from build123d import *

# Parameters (mm, degrees)
EXTRUDE_1_DEPTH         = 12
SKETCH_5_R              = 33
SKETCH_5_R_2            = 10
CUT_EXTRUDE_1_DEPTH     = 349.001436779
CUT_EXTRUDE_2_DEPTH     = 349.001436779
FILLET_1_R              = 2
HOLE_WIZARD_3_2_3_2_1_D = 3.2


with BuildPart() as part:
    # 草图1 → 凸台-拉伸1 (new body)
    with BuildSketch(Plane.XY):
        with BuildLine():
            Line((320, 25), (56.665686266, 25))
            ThreePointArc((56.665686266, 25), (40.770417333, 27.593877763), (26.524363784, 35.106382979))
            ThreePointArc((26.524363784, 35.106382979), (-44, 0), (26.524363784, -35.106382979))
            ThreePointArc((26.524363784, -35.106382979), (40.770417333, -27.593877763), (56.665686266, -25))
            Line((56.665686266, -25), (320, -25))
            ThreePointArc((320, -25), (345, 0), (320, 25))
        make_face()
    extrude(amount=EXTRUDE_1_DEPTH)

    # 草图5 → 切除-拉伸1 (cut, through all)
    with BuildSketch(Plane.XY.offset(12)):
        Circle(SKETCH_5_R)
        with Locations((320, 0)):
            Circle(SKETCH_5_R_2)
    extrude(amount=-CUT_EXTRUDE_1_DEPTH, mode=Mode.SUBTRACT)

    # 草图6 → 切除-拉伸2 (cut, through all)
    with BuildSketch(Plane.XY.offset(12)):
        with BuildLine():
            Line((112.915026221, 15), (82.915026221, -15))
            Line((82.915026221, -15), (72.915026221, -15))
            Line((72.915026221, -15), (52.915026221, -15))
            ThreePointArc((52.915026221, -15), (55, 0), (52.915026221, 15))
            Line((52.915026221, 15), (112.915026221, 15))
        make_face()
        Polygon((97.057161845, -15), (174.604308358, -15), (127.057161845, 15), align=None)
        Polygon((145.797288554, 15), (212.27301577, 15), (193.344435067, -15), align=None)
        Polygon((205.168568427, -15), (224.097149131, 15), (265.168568427, -15), align=None)
        with BuildLine():
            Line((241.050881866, 15), (282.122301163, -15))
            Line((282.122301163, -15), (300, -15))
            ThreePointArc((300, -15), (295, 0), (300, 15))
            Line((300, 15), (241.050881866, 15))
        make_face()
    extrude(amount=-CUT_EXTRUDE_2_DEPTH, mode=Mode.SUBTRACT)

    # 圆角1
    fillet_1_edges = [part.edges().sort_by_distance(p)[0] for p in [
        (97.057161845, -15, 6),
        (127.057161845, 15, 6),
        (174.604308358, -15, 6),
        (82.915026221, -15, 6),
        (52.915026221, -15, 6),
        (52.915026221, 15, 6),
        (112.915026221, 15, 6),
        (193.344435067, -15, 6),
        (145.797288554, 15, 6),
        (212.27301577, 15, 6),
        (241.050881866, 15, 6),
        (300, 15, 6),
        (300, -15, 6),
        (282.122301163, -15, 6),
        (265.168568427, -15, 6),
        (205.168568427, -15, 6),
        (224.097149131, 15, 6),
    ]]
    fillet(fillet_1_edges, radius=FILLET_1_R)

    # Ø3.2 (3.2) 直径孔1 (through all)
    with Locations(Plane(origin=(0, 38.5, 12), x_dir=(1, 0, 0), z_dir=(0, 0, 1))):
        with Locations((0, 0), (-33.341978046, -19.25), (-33.341978046, -57.75), (0, -77), (33.341978046, -57.75), (33.341978046, -19.25)):
            Hole(HOLE_WIZARD_3_2_3_2_1_D / 2)


solid = part.part
Model file for the job. Use its own axes, mm. A direction names the side the tool comes from. Round coordinates to 2 decimals unless told otherwise and drop trailing zeros. Loops run counter-clockwise (first coordinate to the right, second up) from the corner with the lowest first, then second, coordinate; pieces in that order, holes last. Notation, with made-up numbers: (-28.5, 8) -> (7.5, 8) arc R12 cw to (7.5, 29) -> close; hole circle Ø11 at (8, 15). An arc over 180 degrees is marked (long way). Answer as CSV lines item,"result". Start each with the question number.
1) Pin check, flat tips, straight feed: P1, Ø3.5, axis at x = 241.5, z = 3, coming from the -Y side; P2, Ø5, axis at y = 30.5, z = 7.5, coming from the -X side; P3, Ø1, axis at y = 6.5, z = 7.5, coming from the -X side. Stop position of each tip, or through.
2) Probe line 1 along Y through (x, z) = (0, 6.75); line 2 along Y through (x, z) = (159.5, 4); line 3 along Y through (x, z) = (285.5, 9.5). List the from-to ranges inside material, lowest first.
3) Slice it at B-B (x = -18.5). List the corners of the cut face in (y, z), plus the area to 3 significant figures.
4) Slice it at A-A (y = 6.5). State how many separate pieces and enclosed holes the cut face has, plus the area to 3 significant figures.
5) Mould opens along Y. For faces 3 (the face through (134, -15, 6)), 4 (the face through (272, 15, 6)), 5 (the face through (150, 7, 12)), 6 (the face through (186, -25, 6)) say: +Y half, -Y half, draft (parallel to the pull), parting line (faces both ways), or undercut.
6) Tool access for faces 1 (the face through (295, 0, 6)), 2 (the face through (344.994, -0.55, 5.916)): list every direction of +Z, -Z, +X, -X, +Y, -Y with a clear straight run to the whole face (end or side of a thin tool).
Filled in:
1,P1,"stops at y = -25"
1,P2,"stops at x = -33.94"
1,P3,"stops at x = -43.59"
2,line 1,"y = -44 to -40.1, -36.9 to -33, 33 to 36.9, 40.1 to 44"
2,line 2,"y = -25 to -15, -5.47 to 6.35, 15 to 25"
2,line 3,"y = -25 to -15, 15 to 25"
3,outline,"(-39.92, 0) -> (-27.33, 0) -> (-27.33, 12) -> (-39.92, 12) -> close; (27.33, 0) -> (39.92, 0) -> (39.92, 12) -> (27.33, 12) -> close"
3,area,"302 mm2"
4,separate pieces,"8"
4,enclosed holes,"0"
4,area,"1,540 mm2"
5,face 3,"undercut"
5,face 4,"undercut"
5,face 5,"draft"
5,face 6,"-Y half"
6,face 1,"+Z, -Z"
6,face 2,"+Z, -Z, +X"
